The listing builds one solid part. Answer for the finished solid, in the listing's coordinates (mm). Face numbers are marked on the shaded views. A direction names the side the tool comes from. Coordinates: 2 decimals unless noted, no trailing zeros. Order: outer loops, then holes, each group sorted by start corner. A loop starts at its lowest first (then second) coordinate and runs counter-clockwise, first axis right, second up.
```python
from build123d import *

# Parameters (mm, degrees)
F0_W     = 57.15
F0_H     = 57.15
F0_R     = 2.54
F1_DEPTH = 5.08
F2_SIZE  = 2.54
F3_W     = 57.15
F3_H     = 57.15
F4_DEPTH = 90.17
F5_R     = 10.9855
F6_DEPTH = 2.032
F7_R     = 2.921
F8_DEPTH = 21.844


with BuildPart() as f1:
    # F0 (on Top) → F1 (new body)
    with BuildSketch(Plane.XY):
        Rectangle(F0_W, F0_H)
        with Locations((-21.082, -21.082)):
            Circle(F0_R, mode=Mode.SUBTRACT)
        with Locations((21.082, -21.082)):
            Circle(F0_R, mode=Mode.SUBTRACT)
        with Locations((-21.082, 21.082)):
            Circle(F0_R, mode=Mode.SUBTRACT)
        with Locations((21.082, 21.082)):
            Circle(F0_R, mode=Mode.SUBTRACT)
    extrude(amount=F1_DEPTH)

    # F2
    f2_edges = [f1.edges().sort_by_distance(p)[0] for p in [
        (-28.575, 28.575, 2.54),
        (28.575, 28.575, 2.54),
        (28.575, -28.575, 2.54),
        (-28.575, -28.575, 2.54),
    ]]
    chamfer(f2_edges, length=F2_SIZE)

    # F3 (on face) → F4 (join)
    with BuildSketch(Plane(origin=(0, 0, 0), x_dir=(1, 0, 0), z_dir=(0, 0, -1))):
        Rectangle(F3_W, F3_H)
    extrude(amount=F4_DEPTH)

    # F5 (on face) → F6 (join)
    with BuildSketch(Plane.XY.offset(5.08)):
        Circle(F5_R)
    extrude(amount=F6_DEPTH)

    # F7 (on face) → F8 (join)
    with BuildSketch(Plane.XY.offset(7.112)):
        Circle(F7_R)
    extrude(amount=F8_DEPTH)


solid = f1.part
```
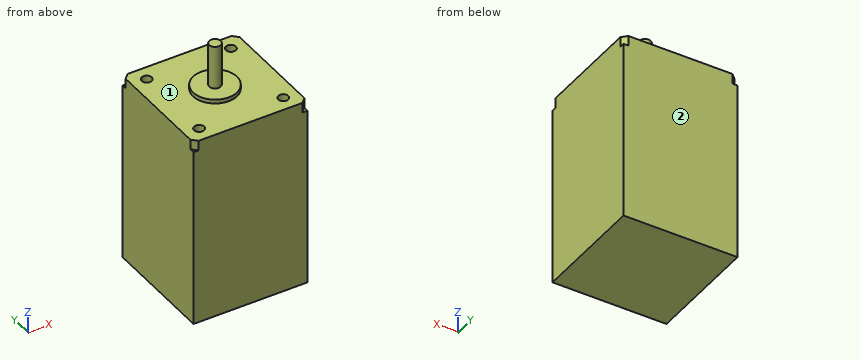
1) Each of these flat-tipped pins is pushed along its axis until it touches: P1, Ø5.5, axis at x = 20.5, y = -20.5, coming from the +Z side; P2, Ø2, axis at x = 4, y = -10, coming from the +Z side; P3, Ø2.5, axis at x = -20, y = -21, coming from the +Z side. Where does it stop, or does it pass through?
2) A cutting plane is placed at C-C, the plane z = 3. Write down the section's boundary in (x, y) (3 decimals), plus the area to 3 significant figures.
3) For the marked faces 1 and 2, determine the directions among +Z, -Z, +X, -X, +Y, -Y from which every point of the face is accessible in a straight line to the end or side of a thin tool.
4) A cutting plane is placed at D-D, the plane y = -12.5. Write down the section's boundary in (x, z) (3 decimals).
5) Straight lines are drawn through the part: probe 1 along Z at (x, y) = (-16, 25.5); probe 2 along Z at (x, y) = (-1, 5). For each, find the intervals that lie inside material, in ascending order.
6) A cutting plane is placed at A-A, the plane y = 0. Write down the section's boundary in (x, z) (1 decimal), plus the area to 3 significant figures.
Working result:
1. P1: stops at z = 5.08
1. P2: stops at z = 7.11
1. P3: stops at z = 0
2. outline: (-28.575, -26.035) - (-26.035, -28.575) - (26.035, -28.575) - (28.575, -26.035) - (28.575, 26.035) - (26.035, 28.575) - (-26.035, 28.575) - (-28.575, 26.035) - close; hole circle Ø5.08 at (-21.082, -21.082); hole circle Ø5.08 at (-21.082, 21.082); hole circle Ø5.08 at (21.082, -21.082); hole circle Ø5.08 at (21.082, 21.082)
2. area: 3,170 mm2
3. face 1: +Z
3. face 2: +Z, -Z, +X, -X, +Y
4. outline: (-28.575, -90.17) - (28.575, -90.17) - (28.575, 5.08) - (-28.575, 5.08) - close
5. probe 1: z = -90.17 to 5.08
5. probe 2: z = -90.17 to 7.11
6. outline: (-28.6, -90.2) - (28.6, -90.2) - (28.6, 5.1) - (11, 5.1) - (11, 7.1) - (2.9, 7.1) - (2.9, 29) - (-2.9, 29) - (-2.9, 7.1) - (-11, 7.1) - (-11, 5.1) - (-28.6, 5.1) - close
6. area: 5,620 mm2
